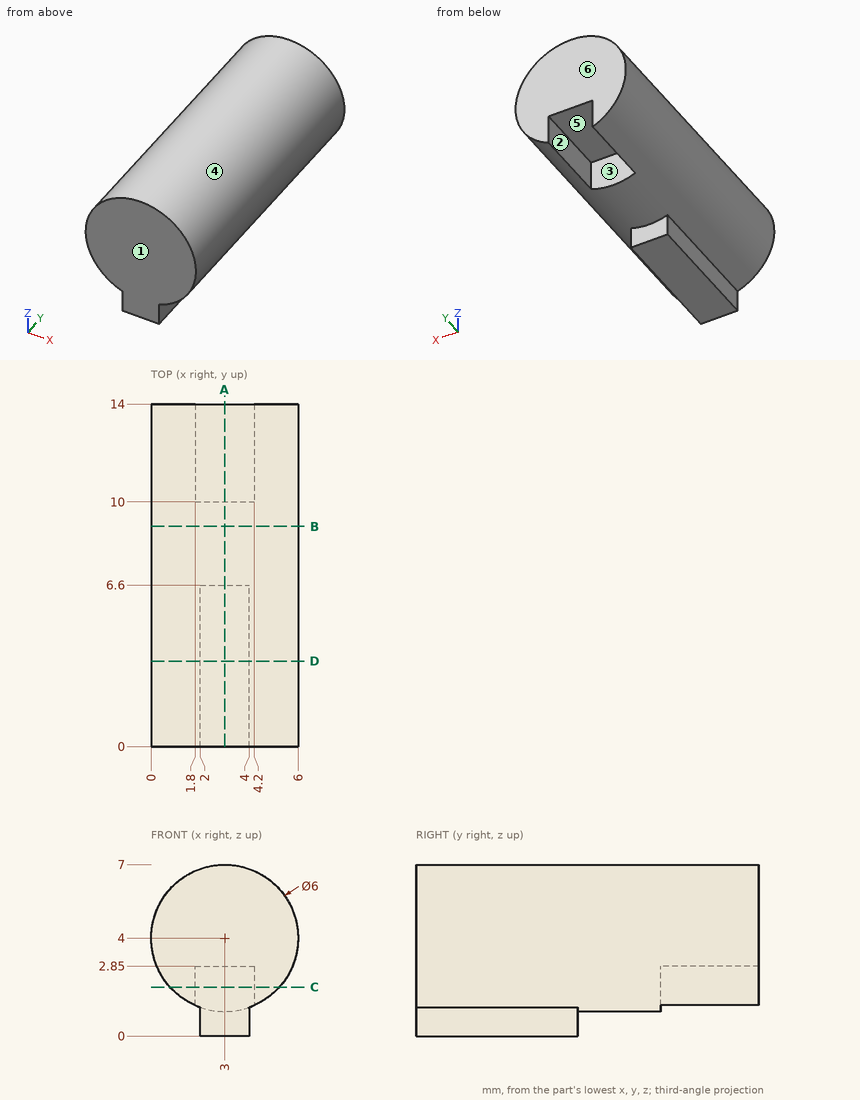
Check sheet for the drawn part. Datum: minimum x, y, z corner. Units: mm. A direction names the side the tool comes from. Coordinates: 2 decimals unless noted, no trailing zeros. Loops run counter-clockwise (first coordinate to the right, second up) from the corner with the lowest first, then second, coordinate; pieces in that order, holes last. Notation, with made-up numbers: (31.5, 6) - (87.5, 6) arc R23 cw to (87.5, 19) - close; hole circle Ø2 at (24.5, 65.5). An arc over 180 degrees is marked (long way). Put each result on its own line as item: value.
Item 1: Scan lines: line 1 along Y through (x, z) = (2.15, 1.75); line 2 along Z through (x, y) = (3, 8.5); line 3 along Y through (x, z) = (2.8, 0.5). Record each from-to range of solid material in increasing order.
Conclusion:
line 1: y = 0 to 10
line 2: z = 1 to 7
line 3: y = 0 to 6.6
Item 2: Gauge pin test, flat ends, axial feed: pin 1 Ø1 at (y, z) = (8.5, 2.5) entering from +X; pin 2 Ø1.8 at (y, z) = (12, 2.5) entering from -X; pin 3 Ø1.8 at (y, z) = (11.5, 2.5) entering from +X. Record the tip position at first contact, or that the pin passes through.
Conclusion:
pin 1: stops at x = 5.83
pin 2: stops at x = 0.06
pin 3: stops at x = 5.94
Item 3: Section check C-C (z = 2). Enter the section's corners in (x, y).
Conclusion:
outline: (0.76, 0) - (5.24, 0) - (5.24, 14) - (4.2, 14) - (4.2, 10) - (1.8, 10) - (1.8, 14) - (0.76, 14) - close
Item 4: Set-up check for the marked faces 1 and 2: record each of +Z, -Z, +X, -X, +Y, -Y from which the full face is reachable in a straight line by a thin tool's end or side.
Conclusion:
face 1: +Z, -Z, +X, -X, -Y
face 2: -Z, +Y
Item 5: Draft check along X on the marked faces 3, 4, 5 and 6. Enter one of: pulls with the +X half, pulls with the -X half, needs draft (parallel to the pull), parting line crosses it, or undercut.
Conclusion:
face 3: undercut
face 4: parting line crosses it
face 5: undercut
face 6: needs draft
Item 6: Section check D-D (y = 3.5). Enter the section's corners in (x, z).
Conclusion:
outline: (2, 0) - (4, 0) - (4, 1.17) arc R3 ccw (long way) to (2, 1.17) - close
Item 7: Section check A-A (x = 3). Enter the section's corners in (y, z).
Conclusion:
outline: (0, 0) - (6.6, 0) - (6.6, 1) - (10, 1) - (10, 2.85) - (14, 2.85) - (14, 7) - (0, 7) - close
Item 8: Section check B-B (y = 9). Enter the section's corners in (x, z), then the cut area to 3 significant figures.
Conclusion:
outline: circle Ø6 at (3, 4)
area: 28.3 mm2
